Geometry: see drawing. Coordinates: mm, zero at the bounding-box minimum. A direction names the side the tool comes from. Coordinates: 2 decimals unless noted, no trailing zeros. Loops run counter-clockwise (first coordinate to the right, second up) from the corner with the lowest first, then second, coordinate; pieces in that order, holes last. Notation, with made-up numbers: (61, 40) - (114, 40) arc R15 ccw to (114, 64) - close; hole circle Ø11 at (-18.75, -31.75). An arc over 180 degrees is marked (long way). Write item = value, one per line. Start each with the question number.
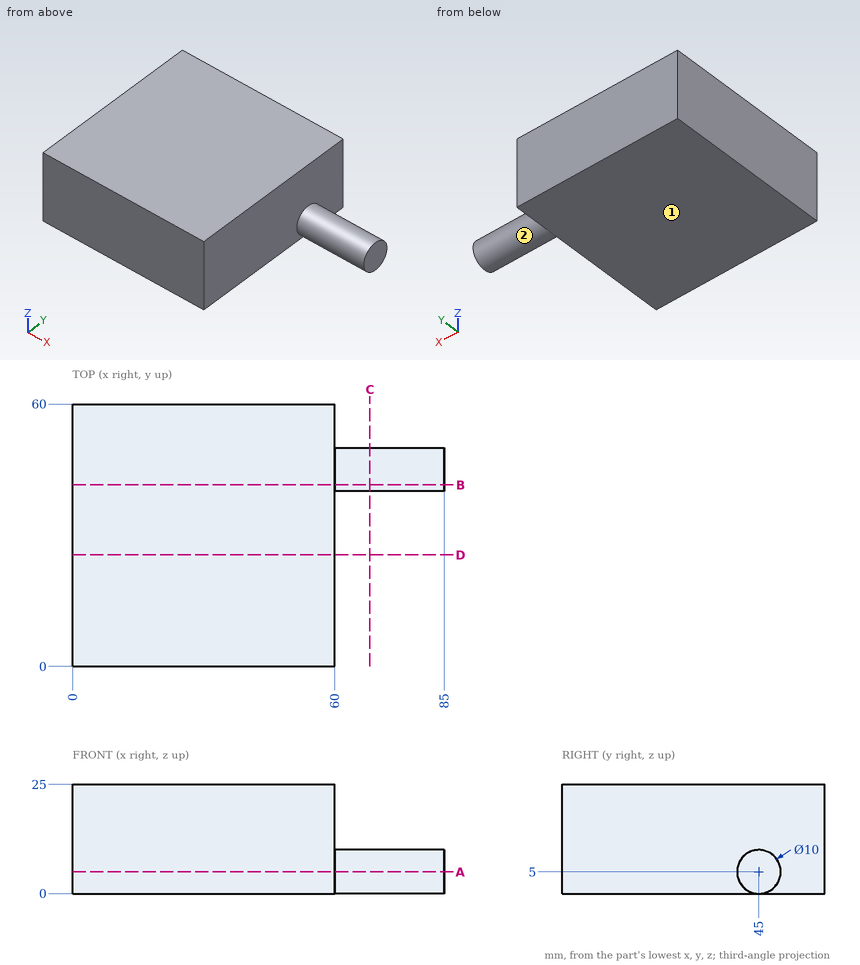
Item 1: First-contact query: pin 1 (4 mm diameter, centred on y = 7.5, z = 19, fed in from +X). Flat tip, straight axial feed; report the tip coordinate or a pass-through.
Item 2: Cut plane B-B (y = 41.5). Return the cut outline in (x, z), then the cut area to 3 significant figures.
Item 3: Material intervals for L1, parallel to X at y = 49, z = 9.75, sorted ascending. Write a range as [from, to].
Item 4: Cut plane A-A (z = 5). Return the cut outline in (x, y), then the cut area to 3 significant figures.
Item 5: Reachability of the marked faces 1 and 2 from +Z, -Z, +X, -X, +Y, -Y: full face, straight path, thin tool, end or side. Return the list, or none.
Item 6: Cut plane D-D (y = 25.5). Return the cut outline in (x, z), then the cut area to 3 significant figures.
Item 7: Cut plane C-C (x = 68). Return the cut outline in (y, z).
Responses:
q1.pin_1 = 60
q2.outline = (0, 0) - (60, 0) - (60, 1.43) - (85, 1.43) - (85, 8.57) - (60, 8.57) - (60, 25) - (0, 25) - close
q2.area = 1,680 mm2
q3.L1 = [0, 60]
q4.outline = (0, 0) - (60, 0) - (60, 40) - (85, 40) - (85, 50) - (60, 50) - (60, 60) - (0, 60) - close
q4.area = 3,850 mm2
q5.face_1 = -Z, +X, -X, +Y, -Y
q5.face_2 = +X
q6.outline = (0, 0) - (60, 0) - (60, 25) - (0, 25) - close
q6.area = 1,500 mm2
q7.outline = circle Ø10 at (45, 5)
